Could you check a few things on this model? Use its own coordinates, in mm. Face numbers are marked on the shaded views. A direction names the side the tool comes from. Coordinates: 2 decimals unless noted, no trailing zeros. Order: outer loops, then holes, each group sorted by start corner. A loop starts at its lowest first (then second) coordinate and runs counter-clockwise, first axis right, second up. Notation, with made-up numbers: (17.5, 11) - (35.5, 11) arc R32 cw to (35.5, 42) - close; hole circle Ø8 at (49.5, 48). An arc over 180 degrees is marked (long way). One line per item, written item: value. Start each with the question number.
from build123d import *

# Parameters (mm, degrees)
SKETCH1_W           = 25.4
SKETCH1_H           = 25.4
SKETCH1_W_2         = 19.05
SKETCH1_H_2         = 19.05
BOSS_EXTRUDE1_DEPTH = 116.84
SKETCH2_R           = 3.175
CUT_EXTRUDE1_DEPTH  = 25.4
SKETCH4_W           = 25.4
SKETCH4_H           = 25.4
SKETCH4_W_2         = 19.05
SKETCH4_H_2         = 19.05
BOSS_EXTRUDE2_DEPTH = 180.848


with BuildPart() as part:
    # Sketch1 → Boss-Extrude1 (new body)
    with BuildSketch(Plane(origin=(0, 0, 0), x_dir=(1, 0, 0), z_dir=(0, 1, 0))):
        with Locations((9.525, 9.525)):
            Rectangle(SKETCH1_W, SKETCH1_H)
        with Locations((9.525, 9.525)):
            Rectangle(SKETCH1_W_2, SKETCH1_H_2, mode=Mode.SUBTRACT)
    boss_extrude1 = extrude(amount=BOSS_EXTRUDE1_DEPTH)

    # Sketch2 → Cut-Extrude1 (cut)
    with BuildSketch(Plane.ZY.offset(3.175)):
        with Locations((-9.525, 15.875)):
            Circle(SKETCH2_R)
        with Locations((-9.525, 38.1)):
            Circle(SKETCH2_R)
    cut_extrude1 = extrude(amount=-CUT_EXTRUDE1_DEPTH, mode=Mode.SUBTRACT)

    # Sketch4 → Boss-Extrude2 (add)
    with BuildSketch(Plane(origin=(22.225, 0, 0), x_dir=(0, 0, -1), z_dir=(1, 0, 0))):
        with Locations((9.525, 104.14)):
            Rectangle(SKETCH4_W, SKETCH4_H)
        with Locations((9.525, 104.14)):
            Rectangle(SKETCH4_W_2, SKETCH4_H_2, mode=Mode.SUBTRACT)
    boss_extrude2 = extrude(amount=BOSS_EXTRUDE2_DEPTH)

    # Mirror2: Boss-Extrude2 across plane
    add(boss_extrude2.mirror(Plane(origin=(203.073, 0, 0), x_dir=(0, 0, 1), z_dir=(1, 0, 0))))

    # Mirror4: Boss-Extrude1, Cut-Extrude1 across plane
    add(boss_extrude1.mirror(Plane(origin=(203.073, 0, 0), x_dir=(0, 0, 1), z_dir=(1, 0, 0))))
    add(cut_extrude1.mirror(Plane(origin=(203.073, 0, 0), x_dir=(0, 0, 1), z_dir=(1, 0, 0))), mode=Mode.SUBTRACT)


solid = part.part
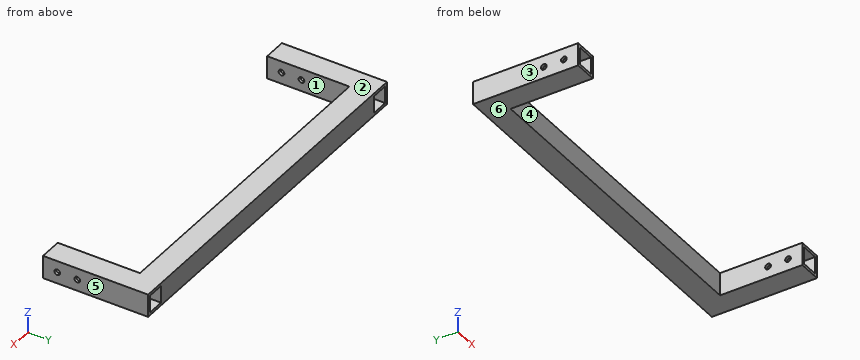
Q1. We'd pull the mould along X, two halves only. Please class the marked faces 3, 4, 5 and 6: +X half, -X half, draft (parallel to the pull), parting line (faces both ways), or undercut.
Q2. I want a section at A-A on x = 232.5. Please give me the cut outline in (y, z) (3 decimals), then the cut area to 3 significant figures.
Q3. I'm going to push flat-ended pins straight in: pin 1 (5.5 mm diameter, centred on y = 15.875, z = -9.525, fed in from +X); pin 2 (15 mm diameter, centred on x = 216.5, z = -5, fed in from -Y). Where does each tip first touch, or does it pass through?
Q4. Which directions (+Z, -Z, +X, -X, +Y, -Y) give clear straight access to the entire face, cutting with the end or side of a thin tool? Please do the marked faces 1 and 2.
Q5. I want a section at B-B on y = 101. Please give me the cut outline in (x, z) (3 decimals).
Q6. If I drill on L1, parallel to X at y = 95, z = -11.5 (3 decimals); L2, parallel to Y at x = 61.5, z = -7 (3 decimals); L3, parallel to Z at x = 145.5, y = 103 (3 decimals), over which ranges is the centre line in solid material (lowest first)?
Values follow:
1. face 3: -X half
1. face 4: undercut
1. face 5: +X half
1. face 6: draft
2. outline: (91.44, -22.225) - (116.84, -22.225) - (116.84, 3.175) - (91.44, 3.175) - close; hole (94.615, -19.05) - (113.665, -19.05) - (113.665, 0) - (94.615, 0) - close
2. area: 282 mm^2
3. pin 1: passes through
3. pin 2: stops at y = 91.44
4. face 1: +Z, -Z, -Y
4. face 2: +Z, +X, -X, +Y, -Y
5. outline: (-3.175, -22.225) - (409.321, -22.225) - (409.321, 3.175) - (-3.175, 3.175) - close; hole (0, -19.05) - (19.05, -19.05) - (19.05, 0) - (0, 0) - close; hole (22.225, -19.05) - (383.921, -19.05) - (383.921, 0) - (22.225, 0) - close; hole (387.096, -19.05) - (406.146, -19.05) - (406.146, 0) - (387.096, 0) - close
6. L1: x = -3.175 to 0, 19.05 to 22.225, 383.921 to 387.096, 406.146 to 409.321
6. L2: y = 91.44 to 94.615, 113.665 to 116.84
6. L3: z = -22.225 to -19.05, 0 to 3.175
